Autodesk Inventor part; units mm, degrees
ref_plane "YZ Plane" through (0, 0, 0) normal (1, 0, 0) x (0, 1, 0)
ref_plane "XZ Plane" through (0, 0, 0) normal (0, 1, 0) x (-1, 0, 0)
ref_plane "XY Plane" through (0, 0, 0) normal (0, 0, 1) x (1, 0, 0)
sketch "Sketch1" plane through (0, 0, 0) normal (0, 1, 0) x (-1, 0, 0)
  line L0 (37.5, 37.5) -> (-37.5, 37.5)
  line L1 (-37.5, 37.5) -> (-37.5, -37.5)
  line L2 (-37.5, -37.5) -> (37.5, -37.5)
  line L3 (37.5, -37.5) -> (37.5, 37.5)
  point P0 (0, 0)
  dimension "d0" = 75
  dimension "d1" = 75
  dimension "d2" = 37.5
  dimension "d3" = 37.5
extrude "Extrusion1" add sketch "Sketch1" along normal blind 19.05
sketch "Sketch3" plane through (0, 19.05, 0) normal (0, 1, 0) x (1, 0, 0)
  line L0 (-37.5, 37.5) -> (-37.5, -37.5)
  line L1 (37.5, 37.5) -> (-37.5, 37.5)
  point P0 (0, 0)
  point P1 (-29.88, 29.88)
  dimension "d27" = 7.62
  dimension "d28" = 7.62
hole "Hole2" at (-29.88, 19.05, -29.88) direction (0, -1, 0) diameter 8.89 depth 11.43
pattern_linear "Rectangular Pattern1" count 2 spacing 59.76 along (1, 0, 0) count 2 spacing 59.76 along (0, 0, 1) of "Hole2"
sketch "Sketch4" plane through (0, 19.05, 0) normal (0, 1, 0) x (1, 0, 0)
  line L0 (37.5, 37.5) -> (-37.5, 37.5)
  point P0 (0, 0)
  point P1 (0, 29.88)
  dimension "d36" = 0
  dimension "d37" = 7.62
hole "Hole3" at (0, 19.05, -29.88) direction (0, -1, 0) diameter 10.16 depth 3.175
mirror "Mirror1" about plane through (0, 0, 0) normal (0, 0, 1) of "Hole3"
sketch "Sketch5" plane through (0, 0, 0) normal (0, -1, 0) x (1, 0, 0)
  point P0 (0, 0)
  point P1 (0, 0)
hole "Hole4" at (0, 0, 0) direction (0, 1, 0) diameter 8.89 depth 11.43
properties part number "antennaTripodMount"
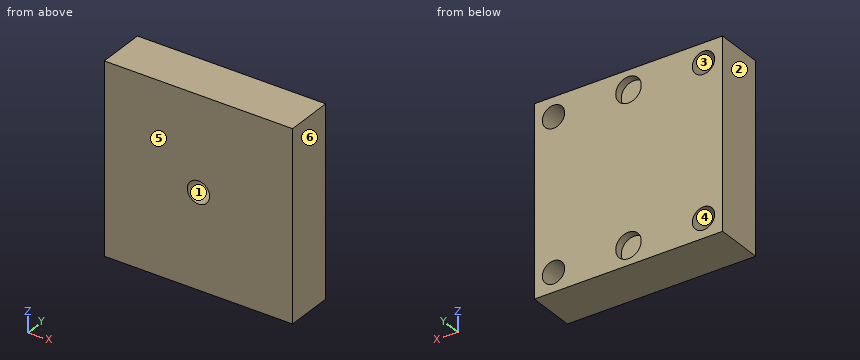
For this review, take the finished solid that the model builds, in its own axes (mm). Face numbers are marked on the shaded views. A direction names the side the tool comes from. Round coordinates to 2 decimals unless told otherwise and drop trailing zeros. Loops run counter-clockwise (first coordinate to the right, second up) from the corner with the lowest first, then second, coordinate; pieces in that order, holes last. Notation, with made-up numbers: (78, -26.5) - (136, -26.5) arc R18 cw to (136, 0.5) - close; hole circle Ø5 at (65.25, -8). An arc over 180 degrees is marked (long way). Use one line per item in the form item = value.
1) We need section A-A on y = 15. Write out the cut boundary in (x, z) (3 decimals), then the cut area to 3 significant figures.
Solutions:
outline = (-37.5, -37.5) - (37.5, -37.5) - (37.5, 37.5) - (-37.5, 37.5) - close; hole circle Ø8.89 at (-29.88, -29.88); hole circle Ø8.89 at (-29.88, 29.88); hole circle Ø8.89 at (29.88, -29.88); hole circle Ø8.89 at (29.88, 29.88)
area = 5,380 mm2
2) Mouldability with a two-part tool opening along X and no side actions: class the marked faces 4, 5 and 6 as pulls with the +X half, pulls with the -X half, needs draft (parallel to the pull), parting line crosses it, or undercut.
Solutions:
face_4 = undercut
face_5 = needs draft
face_6 = pulls with the +X half
3) We need section D-D on z = 29.88. Write out the cut boundary in (x, y) (3 decimals).
Solutions:
outline = (-37.5, 0) - (37.5, 0) - (37.5, 19.05) - (34.325, 19.05) - (34.325, 7.62) - (25.435, 7.62) - (25.435, 19.05) - (5.08, 19.05) - (5.08, 15.875) - (-5.08, 15.875) - (-5.08, 19.05) - (-25.435, 19.05) - (-25.435, 7.62) - (-34.325, 7.62) - (-34.325, 19.05) - (-37.5, 19.05) - close
4) We need section B-B on z = 0. Write out the cut boundary in (x, y) (3 decimals), then the cut area to 3 significant figures.
Solutions:
outline = (-37.5, 0) - (-4.445, 0) - (-4.445, 11.43) - (4.445, 11.43) - (4.445, 0) - (37.5, 0) - (37.5, 19.05) - (-37.5, 19.05) - close
area = 1,330 mm2
5) Wall thickness on probe 1 along Z at (x, y) = (29.88, 14.5) (3 decimals); probe 2 along Z at (x, y) = (0, 16.95); probe 3 along X at (y, z) = (16.75, 29.88) (3 decimals): over which ranges is each line inside the solid? List them lowest first.
Solutions:
probe_1 = -37.5 to -34.325, -25.435 to 25.435, 34.325 to 37.5
probe_2 = -37.5 to -34.96, -24.8 to 24.8, 34.96 to 37.5
probe_3 = -37.5 to -34.325, -25.435 to -5.08, 5.08 to 25.435, 34.325 to 37.5
6) Clearance check with a flat-ended pin moving along its axis: P1, Ø4.5, axis at x = -30, z = -29, coming from the +Y side. State where the tip first meets the part, or that it passes through.
Solutions:
P1 = 7.62
7) We need section C-C on x = 29.88. Write out the cut boundary in (y, z) (3 decimals).
Solutions:
outline = (0, -37.5) - (19.05, -37.5) - (19.05, -34.325) - (7.62, -34.325) - (7.62, -25.435) - (19.05, -25.435) - (19.05, 25.435) - (7.62, 25.435) - (7.62, 34.325) - (19.05, 34.325) - (19.05, 37.5) - (0, 37.5) - close
8) Tool access review of the marked faces 1, 2 and 3: name each direction out of +Z, -Z, +X, -X, +Y, -Y from which nothing blocks a thin tool from reaching the whole face with its end or side.
Solutions:
face_1 = -Y
face_2 = +Z, -Z, -X, +Y, -Y
face_3 = +Y
